Check sheet for the drawn part. Datum: minimum x, y, z corner. Units: mm. A direction names the side the tool comes from. Give positions to 0.01 mm unless a question says otherwise; leave off trailing zeros. Loops run counter-clockwise (first coordinate to the right, second up) from the corner with the lowest first, then second, coordinate; pieces in that order, holes last. Notation, with made-up numbers: M 43.5,69.5 L 92.5,69.5 A31 cw 92.5,101.5 Z; hole C -36,22 d3. An arc over 180 degrees is marked long. Write each question's results on one line, items separated by ' | '. Start each with the question number.
1. Sectioned sample at C-C on x = 8. Record the cut outline in (y, z) (1 decimal).
2. Sectioned sample at D-D on z = 24.75. Record the cut outline in (x, y).
3. Sectioned sample at B-B on y = 14. Record the cut outline in (x, z), and give its area (3 significant figures).
4. Sectioned sample at A-A on z = 10. Record the cut outline in (x, y), and give its area (3 significant figures).
5. Go/stop test with flat-tipped pins: pin 1 (8 mm diameter, centred on x = 14, y = 25.5, fed in from -Z); pin 2 (7 mm diameter, centred on x = 25.5, z = 9, fed in from +Y); pin 3 (2 mm diameter, centred on y = 25, z = 18.5, fed in from +X). Record where each tip stops, or that it passes through.
6. Tool access check on the marked faces 1 and 2. Record the directions out of +Z, -Z, +X, -X, +Y, -Y that give a thin tool (end or side, any length) a straight path to the whole face; none if there is none.
7. Material ranges on line 1 along Y through (x, z) = (12.5, 13.75); line 2 along Z through (x, y) = (17, 6), recorded low to high.
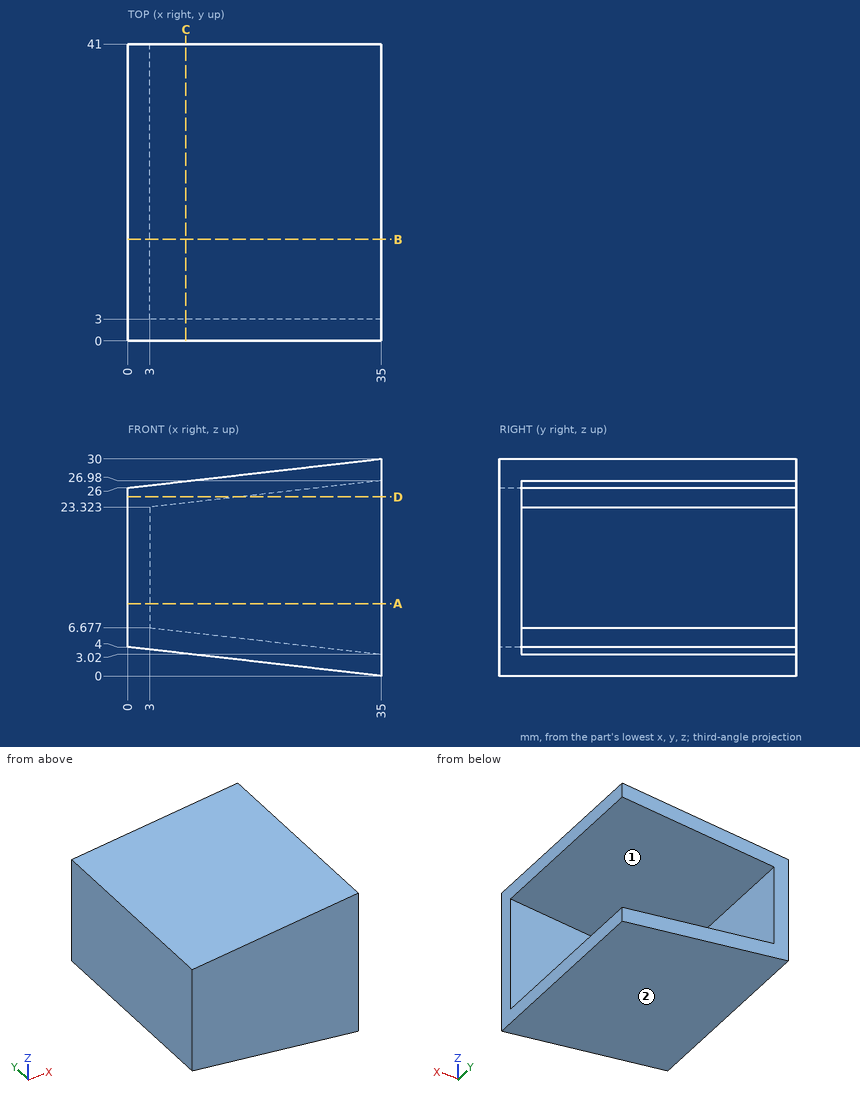
Output values:
1) outline: M 0,3.1 L 41,3.1 L 41,6.1 L 3,6.1 L 3,23.9 L 41,23.9 L 41,26.9 L 0,26.9 Z
2) outline: M 0,0 L 35,0 L 35,3 L 15.48,3 L 15.48,41 L 0,41 Z
3) outline: M 0,4 L 35,0 L 35,3.02 L 3,6.68 L 3,23.32 L 35,26.98 L 35,30 L 0,26 Z | area: 260 mm2
4) outline: M 0,0 L 35,0 L 35,3 L 3,3 L 3,41 L 0,41 Z | area: 219 mm2
5) pin 1: z = 1.94 | pin 2: y = 3 | pin 3: x = 3
6) face 1: +X, +Y | face 2: -Z, -X, +Y, -Y
7) line 1: 0 to 3 | line 2: 2.06 to 5.08, 24.92 to 27.94
